For this review, take the finished solid that the model builds, in its own axes (mm). Give positions to 0.01 mm unless a question says otherwise; leave off trailing zeros. Write each loop counter-clockwise with the first axis right and the second up, starting at its lowest first coordinate (ties: lowest second). Pieces come first, ordered by that corner, then holes. Notation, with made-up numbers: (-31, 17.5) -> (-1, 17.5) arc R14 cw to (-1, 35.5) -> close; hole circle Ø10 at (43, 89). An arc over 180 degrees is marked (long way). Return JSON: item names as keys, results as strings.
Autodesk Inventor part; units mm, degrees
ref_plane "YZ Plane" through (0, 0, 0) normal (1, 0, 0) x (0, 1, 0)
ref_plane "XZ Plane" through (0, 0, 0) normal (0, 1, 0) x (-1, 0, 0)
ref_plane "XY Plane" through (0, 0, 0) normal (0, 0, 1) x (1, 0, 0)
sketch "Sketch1" plane through (0, 0, 0) normal (0, 0, 1) x (1, 0, 0)
  circle A0 centre (0, 0) radius 1.4
  line L0 (5, 16.5227) -> (5, 15.906)
  line L1 (5, -15.906) -> (5, -16.5227)
  line L2 (-5, -16.5227) -> (-5, -15.906)
  line L3 (-5, 15.906) -> (-5, 16.5227)
  arc A1 (-5.6471, 14.9703) -> (-5.6471, -14.9703) centre (0, 0) ccw
  arc A2 (5.6471, -14.9703) -> (5.6471, 14.9703) centre (0, 0) ccw
  arc A3 (-5.6471, 14.9703) -> (-5, 15.906) centre (-6, 15.906) ccw
  arc A4 (-4.2353, 17.4946) -> (-5, 16.5227) centre (-4, 16.5227) ccw
  arc A5 (5, 16.5227) -> (4.2353, 17.4946) centre (4, 16.5227) ccw
  arc A6 (5, 15.906) -> (5.6471, 14.9703) centre (6, 15.906) ccw
  arc A7 (5.6471, -14.9703) -> (5, -15.906) centre (6, -15.906) ccw
  arc A8 (4.2353, -17.4946) -> (5, -16.5227) centre (4, -16.5227) ccw
  arc A9 (-5, -16.5227) -> (-4.2353, -17.4946) centre (-4, -16.5227) ccw
  arc A10 (-5, -15.906) -> (-5.6471, -14.9703) centre (-6, -15.906) ccw
  arc A11 (-1.4959, 16.8897) -> (1.4959, 16.8897) centre (0, 17) ccw
  arc A12 (1.4959, -16.8897) -> (-1.4959, -16.8897) centre (0, -17) ccw
  arc A13 (-4.2353, -17.4946) -> (-2.6399, -17.8054) centre (0, 0) ccw
  arc A14 (2.6399, -17.8054) -> (4.2353, -17.4946) centre (0, 0) ccw
  arc A15 (4.2353, 17.4946) -> (2.6399, 17.8054) centre (0, 0) ccw
  arc A16 (-2.6399, 17.8054) -> (-4.2353, 17.4946) centre (0, 0) ccw
  arc A17 (-1.4959, 16.8897) -> (-2.6399, 17.8054) centre (-2.4932, 16.8162) ccw
  arc A18 (2.6399, 17.8054) -> (1.4959, 16.8897) centre (2.4932, 16.8162) ccw
  arc A19 (-2.6399, -17.8054) -> (-1.4959, -16.8897) centre (-2.4932, -16.8162) ccw
  arc A20 (1.4959, -16.8897) -> (2.6399, -17.8054) centre (2.4932, -16.8162) ccw
  point P0 (5, -17.2916)
  point P1 (-5, -17.2916)
  point P2 (5, 15.1987)
  point P3 (5, -15.1987)
  point P4 (-5, -15.1987)
  point P5 (-5, 15.1987)
  point P6 (-5, 17.2916)
  point P7 (5, 17.2916)
  dimension "d3" = 2.8
  dimension "d9" = 1
  dimension "d12" = 16
  dimension "d13" = 16
  dimension "d14" = 10
  dimension "d15" = 10
  dimension "d16" = 5
  dimension "d17" = 5
  dimension "d18" = 3
  dimension "d19" = 17
  dimension "d20" = 3
  dimension "d21" = 17
  dimension "d22" = 1
extrude "Extrusion1" add sketch "Sketch1" along normal blind 3
properties part number "Front Outer Endcap"
1. Add section B-B, the plane y = 0. State the section outline as (x, z) points, plus the area to 3 significant figures.
Results found:
{"outline": "(-16, 0) -> (-1.4, 0) -> (-1.4, 3) -> (-16, 3) -> close; (1.4, 0) -> (16, 0) -> (16, 3) -> (1.4, 3) -> close", "area": "87.6 mm²"}
2. To check wall thickness, follow probe 1 along Y at (x, z) = (-8.5, 1); probe 2 along X at (y, z) = (-14.5, 1.7); probe 3 along Y at (x, z) = (1, 2.45). State the ranges of each line that lie inside material, in increasing order.
Results found:
{"probe 1": "y = -13.56 to 13.56", "probe 2": "x = -6.76 to 6.76", "probe 3": "y = -15.88 to -0.98, 0.98 to 15.88"}
3. Add section A-A, the plane x = 0. State the section outline as (y, z) points, plus the area to 3 significant figures.
Results found:
{"outline": "(-15.5, 0) -> (-1.4, 0) -> (-1.4, 3) -> (-15.5, 3) -> close; (1.4, 0) -> (15.5, 0) -> (15.5, 3) -> (1.4, 3) -> close", "area": "84.6 mm²"}
4. Add section C-C, the plane z = 0.5. State the section outline as (x, y) points, plus the area to 3 significant figures.
Results found:
{"outline": "(-5.65, -14.97) arc R1 cw to (-5, -15.91) -> (-5, -16.52) arc R1 ccw to (-4.24, -17.49) arc R18.03 ccw to (-2.64, -17.81) arc R1 ccw to (-1.5, -16.89) arc R1.5 cw to (1.5, -16.89) arc R1 ccw to (2.64, -17.81) arc R17.97 ccw to (4.24, -17.49) arc R1 ccw to (5, -16.52) -> (5, -15.91) arc R1 cw to (5.65, -14.97) arc R16 ccw to (5.65, 14.97) arc R1 cw to (5, 15.91) -> (5, 16.52) arc R1 ccw to (4.24, 17.49) arc R18.03 ccw to (2.64, 17.81) arc R1 ccw to (1.5, 16.89) arc R1.5 cw to (-1.5, 16.89) arc R1 ccw to (-2.64, 17.81) arc R17.97 ccw to (-4.24, 17.49) arc R1 ccw to (-5, 16.52) -> (-5, 15.91) arc R1 cw to (-5.65, 14.97) arc R16 ccw to start; hole circle Ø2.8 at (0, 0)", "area": "825 mm²"}
5. For pin 1 (0.5 mm diameter, centred on y = -16, z = 1.5, fed in from +X); pin 2 (2.5 mm diameter, centred on x = 0, y = 0, fed in from +Z), all flat-tipped, find the tip position at first contact; note any pin that passes through.
Results found:
{"pin 1": "stops at x = 5.01", "pin 2": "passes through"}
6. Add section D-D, the plane x = -14. State the section outline as (y, z) points.
Results found:
{"outline": "(-7.75, 0) -> (7.75, 0) -> (7.75, 3) -> (-7.75, 3) -> close"}
7. The part is to be moulded in two halves that separate along X. For faces 1 (the cylindrical face through (-4.792, 17.134, 1.479)), 2 (the cylindrical face through (5.173, -15.344, 1.479)), 3 (the cylindrical face through (0, -15.5, 1.5)), say which applies: +X half, -X half, draft (parallel to the pull), parting line (faces both ways), or undercut.
Results found:
{"face 1": "-X half", "face 2": "+X half", "face 3": "undercut"}
